from build123d import *

# Parameters (mm, degrees)
SKETCH1_R           = 15
BOSS_EXTRUDE1_DEPTH = 10
SKETCH2_R           = 15
BOSS_EXTRUDE2_DEPTH = 10
SKETCH3_R           = 15
BOSS_EXTRUDE3_DEPTH = 10
SKETCH4_R           = 5
CUT_EXTRUDE1_DEPTH  = 36


with BuildPart() as part:
    # Sketch1 → Boss-Extrude1 (new body)
    with BuildSketch(Plane(origin=(0, 0, 0), x_dir=(0, 0, -1), z_dir=(1, 0, 0))):
        with BuildLine():
            ThreePointArc((20, 15), (-25, 0), (20, -15))
            ThreePointArc((20, -15), (40, -5), (60, -15))
            ThreePointArc((60, -15), (105, 0), (60, 15))
            ThreePointArc((60, 15), (40, 5), (20, 15))
        make_face()
        Circle(SKETCH1_R, mode=Mode.SUBTRACT)
        with Locations((80, 0)):
            Circle(SKETCH1_R, mode=Mode.SUBTRACT)
    extrude(amount=BOSS_EXTRUDE1_DEPTH)

    # Sketch2 → Boss-Extrude2 (add)
    with BuildSketch(Plane.ZY):
        Circle(SKETCH2_R)
    extrude(amount=-BOSS_EXTRUDE2_DEPTH)

    # Sketch3 → Boss-Extrude3 (add)
    with BuildSketch(Plane.ZY):
        Circle(SKETCH3_R)
    extrude(amount=BOSS_EXTRUDE3_DEPTH)

    # Sketch4 → Cut-Extrude1 (cut)
    with BuildSketch(Plane.ZY.offset(10)):
        Circle(SKETCH4_R)
    extrude(amount=-CUT_EXTRUDE1_DEPTH, mode=Mode.SUBTRACT)


solid = part.part
Part model, mm, in its own coordinate system. Coordinates: 2 decimals unless noted, no trailing zeros. Loops run counter-clockwise (first coordinate to the right, second up) from the corner with the lowest first, then second, coordinate; pieces in that order, holes last. Notation, with made-up numbers: M 74,-13 L 89,-13 A27 ccw 89,9 Z; hole C 49,2.25 d9. An arc over 180 degrees is marked long. Use a Markdown table: item, result. Add a question column.
Q1. Cut at A-A (z = 0). Write the cut outline in (x, y).
Q2. Pin check, flat tips, straight feed: P1, Ø3, axis at x = 3.5, y = -15, coming from the -Z side; P2, Ø11.5, axis at y = 0, z = 0, coming from the -X side; P3, Ø12, axis at x = 3.5, y = 17, coming from the -Z side; P4, Ø2, axis at x = -8, y = -17, coming from the -Z side. Stop position of each tip, or through.
Q3. Cut at C-C (x = -1.25). Write the cut outline in (y, z).
Q4. Cut at D-D (z = -80). Write the cut outline in (x, y), and give its area (3 significant figures).
Q5. Probe L1, parallel to Y at x = 2.5, z = -80; L2, parallel to Y at x = 4.75, z = 0; L3, parallel to Z at x = 6.5, y = -8. List the from-to ranges inside material, lowest first.
Q6. Mould opens along Y. For faces 1 (the flat face through (10, 0, -39)), 2 (the cylindrical face through (-4.93, 0.66, -14.985)), 3 (the cylindrical face through (-0.14, -4.88, -1.08)) say: +Y half, -Y half, draft (parallel to the pull), parting line (faces both ways), or undercut.
Q7. Cut at B-B (y = 0). Write the cut outline in (x, z), and give its area (3 significant figures).
Worked out:
| question | item | result |
|---|---|---|
| 1 | outline | M -10,-15 L 0,-15 L 0,-25 L 10,-25 L 10,-5 L -10,-5 Z; M -10,5 L 10,5 L 10,25 L 0,25 L 0,15 L -10,15 Z |
| 2 | P1 | stops at z = -101.04 |
| 2 | P2 | stops at x = -10 |
| 2 | P3 | stops at z = -102.45 |
| 2 | P4 | passes through |
| 3 | outline | C 0,0 d30; hole C 0,0 d10 |
| 4 | outline | M 0,-25 L 10,-25 L 10,-15 L 0,-15 Z; M 0,15 L 10,15 L 10,25 L 0,25 Z |
| 4 | area | 200 mm2 |
| 5 | L1 | y = -25 to -15, 15 to 25 |
| 5 | L2 | y = -25 to -5, 5 to 25 |
| 5 | L3 | z = -103.69 to -92.69, -67.31 to -51.87, -28.13 to 23.69 |
| 6 | face 1 | draft |
| 6 | face 2 | parting line |
| 6 | face 3 | undercut |
| 7 | outline | M -10,-15 L 0,-15 L 0,-65 L 10,-65 L 10,-5 L -10,-5 Z; M -10,5 L 10,5 L 10,25 L 0,25 L 0,15 L -10,15 Z; M 0,-105 L 10,-105 L 10,-95 L 0,-95 Z |
| 7 | area | 1,100 mm2 |
